from build123d import *

# Parameters (mm, degrees)
SKETCH001_R       = 108
SKETCH001_R_2     = 86.75
SKETCH001_R_3     = 2.5
PAD_DEPTH         = 10
SKETCH_R          = 1.5625
POCKET_DEPTH      = 10.001
POCKET_DEPTH_BACK = 0.001


with BuildPart() as part:
    # Sketch001 → Pad (new body)
    with BuildSketch(Plane(origin=(0, 0, 0), x_dir=(1, 0, 0), z_dir=(0, 0, -1))):
        Circle(SKETCH001_R)
        Circle(SKETCH001_R_2, mode=Mode.SUBTRACT)
        with Locations((38.651027, 93.311833)):
            Circle(SKETCH001_R_3, mode=Mode.SUBTRACT)
        with Locations((93.311833, 38.651027)):
            Circle(SKETCH001_R_3, mode=Mode.SUBTRACT)
        with Locations((93.311833, -38.651027)):
            Circle(SKETCH001_R_3, mode=Mode.SUBTRACT)
        with Locations((38.651027, -93.311833)):
            Circle(SKETCH001_R_3, mode=Mode.SUBTRACT)
        with Locations((-38.651027, 93.311833)):
            Circle(SKETCH001_R_3, mode=Mode.SUBTRACT)
        with Locations((-93.311833, 38.651027)):
            Circle(SKETCH001_R_3, mode=Mode.SUBTRACT)
        with Locations((-93.311833, -38.651027)):
            Circle(SKETCH001_R_3, mode=Mode.SUBTRACT)
        with Locations((-38.651027, -93.311833)):
            Circle(SKETCH001_R_3, mode=Mode.SUBTRACT)
    extrude(amount=PAD_DEPTH)

    # Sketch → Pocket (cut, two sides)
    with BuildSketch(Plane.XY) as pocket_sk:
        with Locations((64.346717, 64.346717)):
            Circle(SKETCH_R)
        with Locations((0, 91)):
            Circle(SKETCH_R)
        with Locations((91, 0)):
            Circle(SKETCH_R)
        with Locations((64.346717, -64.346717)):
            Circle(SKETCH_R)
        with Locations((0, -91)):
            Circle(SKETCH_R)
        with Locations((-91, 0)):
            Circle(SKETCH_R)
        with Locations((-64.346717, -64.346717)):
            Circle(SKETCH_R)
        with Locations((-64.346717, 64.346717)):
            Circle(SKETCH_R)
    extrude(amount=-POCKET_DEPTH, mode=Mode.SUBTRACT)
    extrude(pocket_sk.sketch, amount=POCKET_DEPTH_BACK, mode=Mode.SUBTRACT)


solid = part.part
Geometry: final body of the model. Coordinates: model frame, mm. Give positions to 0.01 mm unless a question says otherwise; leave off trailing zeros. Write each loop counter-clockwise with the first axis right and the second up, starting at its lowest first coordinate (ties: lowest second). Pieces come first, ordered by that corner, then holes.
(1) Ray query, line 1 (Y direction, x = 0, z = -5); line 2 (X direction, y = 95, z = -1.25); line 3 (X direction, y = 7, z = -3.25). Return the intervals inside material, ascending.
(2) First-contact query: P1, Ø2.5, axis at x = 91, y = 0, coming from the -Z side; P2, Ø6.5, axis at x = 38.65, y = 93.31, coming from the +Z side; P3, Ø6, axis at y = -47, z = -6.5, coming from the +X side; P4, Ø3, axis at y = -5, z = -3.5, coming from the -X side. Flat tips, straight axial feed; report the tip coordinate or a pass-through.
(3) Cut plane C-C, the plane z = -7.5. Give the number of separate pieces and of enclosed holes in the cut face, then the cut area to 3 significant figures.
(4) Cut plane B-B, the plane y = -75. Return loops of the section in (x, z), then the cut area to 3 significant figures.
(5) Mould query, pull axis X, two halves, no side actions, for faces 1 (the cylindrical face through (-38.976, 90.833, -4.93)), 2 (the flat face through (-81, -33, 0)), 3 (the cylindrical face through (-23.412, 105.432, -4.93)). Classes: released by +X, released by -X, zero draft, split by the parting line, or undercut.
(6) Cut plane A-A, the plane x = 7.5. Return loops of the section in (y, z), then the cut area to 3 significant figures.
Values follow:
1. line 1: y = -108 to -92.56, -89.44 to -86.75, 86.75 to 89.44, 92.56 to 108
1. line 2: x = -51.37 to -40.49, -36.81 to 36.81, 40.49 to 51.37
1. line 3: x = -107.77 to -86.47, 86.47 to 107.77
2. P1: passes through
2. P2: stops at z = 0
2. P3: stops at x = 98.63
2. P4: stops at x = -107.94
3. separate pieces: 1
3. enclosed holes: 17
3. area: 12,800 mm2
4. outline: (-77.71, -10) - (-43.6, -10) - (-43.6, 0) - (-77.71, 0) - close; (43.6, -10) - (77.71, -10) - (77.71, 0) - (43.6, 0) - close
4. area: 682 mm2
5. face 1: undercut
5. face 2: zero draft
5. face 3: split by the parting line
6. outline: (-107.74, -10) - (-86.43, -10) - (-86.43, 0) - (-107.74, 0) - close; (86.43, -10) - (107.74, -10) - (107.74, 0) - (86.43, 0) - close
6. area: 426 mm2
